Part model, mm, in its own coordinate system. A direction names the side the tool comes from. Round coordinates to 2 decimals unless told otherwise and drop trailing zeros. Loops run counter-clockwise (first coordinate to the right, second up) from the corner with the lowest first, then second, coordinate; pieces in that order, holes last. Notation, with made-up numbers: (2.25, -34) -> (33.25, -34) arc R24 ccw to (33.25, -16) -> close; hole circle Ø3 at (56.5, 44.5). An arc over 180 degrees is marked (long way). Answer as CSV lines item,"result".
from build123d import *

# Parameters (mm, degrees)
SKETCH_1_W                       = 100
SKETCH_1_H                       = 50
EXTRUDE_1_DEPTH                  = 5
SKETCH_2_W                       = 5
SKETCH_2_H                       = 20
EXTRUDE_2_DEPTH                  = 5
SKETCH_3_W                       = 20
SKETCH_3_H                       = 5
EXTRUDE_3_DEPTH                  = 5
MIRROR_3_COPY_1_SKETCH_W         = 20
MIRROR_3_COPY_1_SKETCH_H         = 5
MIRROR_3_COPY_1_DEPTH            = 5
PATTERN_LINEAR_2_COUNT           = 2
PATTERN_LINEAR_2_PITCH           = 40
PATTERN_LINEAR_2_COPY_1_SKETCH_W = 5
PATTERN_LINEAR_2_COPY_1_SKETCH_H = 20
PATTERN_LINEAR_2_COPY_1_DEPTH    = 5


with BuildPart() as part:
    # 스케치1 → 보스-돌출1 (new body)
    with BuildSketch(Plane.XY):
        Rectangle(SKETCH_1_W, SKETCH_1_H)
    extrude(amount=EXTRUDE_1_DEPTH)

    # 스케치2 → 보스-돌출2 (add)
    with BuildSketch(Plane.XY.offset(5)):
        with Locations((52.5, -20)):
            Rectangle(SKETCH_2_W, SKETCH_2_H)
    extrude_2 = extrude(amount=-EXTRUDE_2_DEPTH)

    # 대칭 복사1: 보스-돌출2 across plane
    add(extrude_2.mirror(Plane(origin=(0, 0, 0), x_dir=(0, 0, 1), z_dir=(1, 0, 0))))

    # 스케치3 → 보스-돌출3 (add)
    with BuildSketch(Plane.XY.offset(5)):
        with Locations((20, 27.5)):
            Rectangle(SKETCH_3_W, SKETCH_3_H)
    extrude_3 = extrude(amount=-EXTRUDE_3_DEPTH)

    # 대칭 복사2: 보스-돌출3 across plane
    add(extrude_3.mirror(Plane(origin=(0, 0, 0), x_dir=(0, 0, 1), z_dir=(1, 0, 0))))

    # 대칭 복사3: 보스-돌출3 across plane
    add(extrude_3.mirror(Plane.ZX))

    # 대칭 복사3 copy 1 sketch → 대칭 복사3 copy 1 (add)
    with BuildSketch(Plane(origin=(0, 0, 5), x_dir=(-1, 0, 0), z_dir=(0, 0, 1))):
        with Locations((20, 27.5)):
            Rectangle(MIRROR_3_COPY_1_SKETCH_W, MIRROR_3_COPY_1_SKETCH_H)
    extrude(amount=-MIRROR_3_COPY_1_DEPTH)

    # 선형 패턴2: 보스-돌출2 ×2
    with Locations(*[(0, i * PATTERN_LINEAR_2_PITCH, 0) for i in range(1, PATTERN_LINEAR_2_COUNT)]):
        add(extrude_2)

    # 선형 패턴2 copy 1 sketch → 선형 패턴2 copy 1 (add)
    with BuildSketch(Plane(origin=(0, 40, 5), x_dir=(-1, 0, 0), z_dir=(0, 0, 1))):
        with Locations((52.5, 20)):
            Rectangle(PATTERN_LINEAR_2_COPY_1_SKETCH_W, PATTERN_LINEAR_2_COPY_1_SKETCH_H)
    extrude(amount=-PATTERN_LINEAR_2_COPY_1_DEPTH)


solid = part.part
Q1. Drill centre lines: line 1 along X through (y, z) = (-26, 4.65); line 2 along Y through (x, z) = (8, 2.45); line 3 along X through (y, z) = (5.5, 3.6). Where is each one in solid material? Low to high.
Geometry results:
line 1,"-55 to -50, -30 to -10, 10 to 30, 50 to 55"
line 2,"-25 to 25"
line 3,"-50 to 50"
Q2. Drop flat-ended pins along their axis: P1, Ø2.5, axis at x = -0.5, z = 3.5, coming from the +Y side; P2, Ø1.5, axis at y = -1, z = 1.5, coming from the -X side. Give the stop position or say it passes through.
Geometry results:
P1,"y = 25"
P2,"x = -50"
Q3. Which spindle directions (+Z, -Z, +X, -X, +Y, -Y) get a long thin tool onto all of the face, cutting with end or side? Do faces 1 (the face through (50, 0, 2)), 2 (the face through (-50, -28, 3)), 3 (the face through (40, 25, 2)). Say none if no direction does.
Geometry results:
face 1,"+Z, -Z, +X"
face 2,"+Z, -Z, -Y"
face 3,"+Z, -Z, +Y"
Q4. Saw through at B-B, the plane x = -2. Write the cut outline in (y, z), then the cut area to 3 significant figures.
Geometry results:
outline,"(-25, 0) -> (25, 0) -> (25, 5) -> (-25, 5) -> close"
area,"250 mm2"
Q5. Two-plate mould, pull along Y, no slides. Class faces 4 (the face through (-52, 10, 3)), 5 (the face through (0, 25, 2)), 6 (the face through (-30, 27, 3)), 7 (the face through (-20, -30, 3)): pulls with the +Y half, pulls with the -Y half, needs draft (parallel to the pull), parting line crosses it, or undercut.
Geometry results:
face 4,"undercut"
face 5,"pulls with the +Y half"
face 6,"needs draft"
face 7,"pulls with the -Y half"
Q6. Saw through at C-C, the plane y = 3. Write the cut outline in (x, z).
Geometry results:
outline,"(-50, 0) -> (50, 0) -> (50, 5) -> (-50, 5) -> close"
Q7. Saw through at A-A, the plane y = 26.5. Write the cut outline in (x, z), then the cut area to 3 significant figures.
Geometry results:
outline,"(-55, 0) -> (-50, 0) -> (-50, 5) -> (-55, 5) -> close; (-30, 0) -> (-10, 0) -> (-10, 5) -> (-30, 5) -> close; (10, 0) -> (30, 0) -> (30, 5) -> (10, 5) -> close; (50, 0) -> (55, 0) -> (55, 5) -> (50, 5) -> close"
area,"250 mm2"
